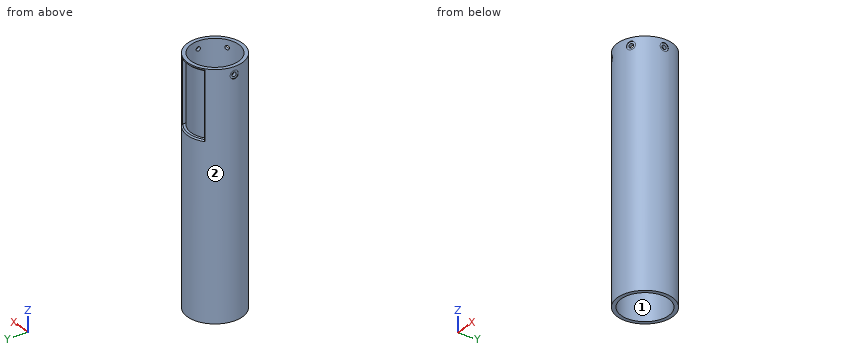
Autodesk Inventor part; units mm, degrees
ref_plane "Plan de construction2" through (22, 0, 96) normal (1, 0, 0) x (0, 1, 0)
ref_plane "Plan de construction3" through (0, -22, 96) normal (0, 1, 0) x (-1, 0, 0)
ref_plane "XY Plane" through (0, 0, 0) normal (0, 0, 1) x (1, 0, 0)
sketch "Esquisse1" plane through (0, 0, 0) normal (1, 0, 0) x (0, 1, 0)
  line L0 (0, 0) -> (0, 594.5025)
  line L1 (22, 0) -> (22, 192)
  line L2 (19, 0) -> (19, 192)
  line L3 (22, 192) -> (19, 192)
  line L4 (22, 0) -> (19, 0)
  dimension "d0" = 38
  dimension "d3" = 3
  dimension "d58" = 192
revolve "Révolution1" add sketch "Esquisse1" angle 360 about axis through (0, 0, 0) along (0, 0, 1)
sketch "Esquisse3" plane through (0, 0, 0) normal (0, 1, 0) x (-1, 0, 0)
  line L0 (-19, 192) -> (19, 192)
  line L1 (12.5, 190) -> (-12.5, 190)
  line L2 (-12.5, 190) -> (-12.5, 138)
  line L3 (-12.5, 138) -> (12.5, 138)
  line L4 (12.5, 138) -> (12.5, 190)
  point P0 (0, 0)
  point P1 (0, 190)
  point P2 (0, 192)
  dimension "d108" = 52
  dimension "d109" = 2
  dimension "d110" = 25
extrude "Extrusion2" cut sketch "Esquisse3" along normal up to surface
ref_plane "Plan de construction2" through (22, 0, 96) normal (1, 0, 0) x (0, 1, 0)
sketch "Esquisse4" plane through (22, 0, 96) normal (1, 0, 0) x (0, 1, 0)
  line L0 (-22, 96) -> (22, 96)
  point P0 (0, -96)
  point P1 (0, 90)
  dimension "d24" = 6
hole "Perçage1" at (22, 0, 186) direction (-1, 0, 0) diameter 3.4 depth 8 counterbore diameter 6.5 counterbore depth 0.5
pattern_circular "Réseau circulaire2" count 4 over 180 about axis through (0, 0, -10) along (0, 0, -1) of "Perçage1"
chamfer "Chanfrein2" distance 1 angle 45 6 edges at (-12.5, 18.1039, 164) (-6.5466, 21.0034, 138) (6.5466, 21.0034, 138) (12.5, 18.1039, 164) (-6.5466, 21.0034, 190) (6.5466, 21.0034, 190)
ref_plane "Plan de construction3" through (0, -22, 96) normal (0, 1, 0) x (-1, 0, 0)
thread "Filetage3"
properties part number "reservoir_guide"
Work out the finished part from the listing and answer in its coordinate system (mm). Face numbers are marked on the shaded views. Give positions to 0.01 mm unless a question says otherwise; leave off trailing zeros. Write each loop counter-clockwise with the first axis right and the second up, starting at its lowest first coordinate (ties: lowest second). Pieces come first, ordered by that corner, then holes. Notation, with made-up numbers: M -22,66 L 22,66 A24 cw 22,81 Z; hole C 17.25,88 d1. An arc over 180 degrees is marked long. Answer as CSV lines item,"result".
Q1. The mould has two halves that part along X. Classify the marked faces 1 and 2: +X half, -X half, draft (parallel to the pull), parting line (faces both ways), or undercut.
A:
face 1,"undercut"
face 2,"parting line"
Q2. Given P1, Ø4, axis at y = 0, z = 186, coming from the -X side; P2, Ø7.5, axis at x = 2.5, y = 16.5, coming from the +Z side; P3, Ø3, axis at y = 0, z = 186, coming from the +X side; P4, Ø2, axis at x = -17, z = 65, coming from the +Y side, each flat-ended and moving along its own axis, determine where each tip first touches the part or whether it passes through.
A:
P1,"stops at x = -21.5"
P2,"stops at z = 192"
P3,"passes through"
P4,"stops at y = 15.1"
Q3. A cutting plane is placed at A-A on y = 0. Write down the section's boundary in (x, z).
A:
outline,"M -22,0 L -19,0 L -19,184.3 L -21.5,184.3 L -21.5,182.75 L -22,182.75 Z; M -22,189.25 L -21.5,189.25 L -21.5,187.7 L -19,187.7 L -19,192 L -22,192 Z; M 19,0 L 22,0 L 22,182.75 L 21.5,182.75 L 21.5,184.3 L 19,184.3 Z; M 19,187.7 L 21.5,187.7 L 21.5,189.25 L 22,189.25 L 22,192 L 19,192 Z"
Q4. A cutting plane is placed at B-B on x = 0. Write down the section's boundary in (y, z).
A:
outline,"M -22,0 L -19,0 L -19,192 L -22,192 Z; M 19,0 L 22,0 L 22,137 L 21,138 L 19,138 Z; M 19,190 L 21,190 L 22,191 L 22,192 L 19,192 Z"
Q5. Find the intervals of material crossed by probe 1 along Z at (x, y) = (-21, 0); probe 2 along Y at (x, z) = (0, 58); probe 3 along Z at (x, y) = (21.8, 0), in increasing order. Write a range as [from, to].
A:
probe 1,"z = [0, 184.3], [187.7, 192]"
probe 2,"y = [-22, -19], [19, 22]"
probe 3,"z = [0, 182.75], [189.25, 192]"
Q6. A cutting plane is placed at D-D on z = 62. Write down the section's boundary in (x, y), plus the area to 3 significant figures.
A:
outline,"C 0,0 d44; hole C 0,0 d38"
area,"386 mm²"
Q7. A cutting plane is placed at C-C on z = 148. Write down the section's boundary in (x, y).
A:
outline,"M -13.31,17.52 A22 ccw long 13.31,17.52 L 12.5,17.1 L 12.5,14.31 A19 cw long -12.5,14.31 L -12.5,17.1 Z"
